Input: part model. Units: mm. Frame: model coordinates. Face numbers are marked on the shaded views. A direction names the side the tool comes from. Round coordinates to 2 decimals unless told otherwise and drop trailing zeros. Order: outer loops, then holes, each group sorted by start corner. A loop starts at its lowest first (then second) coordinate and runs counter-clockwise, first axis right, second up. Notation, with made-up numbers: (33.5, -38) -> (41.5, -38) arc R6 cw to (41.5, -30) -> close; hole circle Ø6 at (6, -32.5). An arc over 180 degrees is marked (long way). Use a Markdown table: item, result.
from build123d import *

# Parameters (mm, degrees)
SKETCH_1_W      = 23
SKETCH_1_H      = 15
SKETCH_1_R      = 1.6
EXTRUDE_1_DEPTH = 1.6
SKETCH_2_W      = 8
SKETCH_2_H      = 4
EXTRUDE_2_DEPTH = 1.8
SKETCH_4_W      = 8
SKETCH_4_H      = 1.25
EXTRUDE_3_DEPTH = 1.6
SKETCH_5_W      = 8
SKETCH_5_H      = 2.2
EXTRUDE_4_DEPTH = 1.2
FILLET_1_R      = 0.8
FILLET_2_R      = 3


with BuildPart() as part:
    # 草图1 → 凸台-拉伸1 (new body)
    with BuildSketch(Plane.XY):
        Rectangle(SKETCH_1_W, SKETCH_1_H)
        with Locations((-8, 0)):
            Circle(SKETCH_1_R, mode=Mode.SUBTRACT)
    extrude(amount=EXTRUDE_1_DEPTH)

    # 草图2 → 凸台-拉伸2 (add)
    with BuildSketch(Plane(origin=(0, 0, 0), x_dir=(-1, 0, 0), z_dir=(0, 0, -1))):
        with Locations((-0.023575702, 5.5)):
            Rectangle(SKETCH_2_W, SKETCH_2_H)
        with Locations((-0.023575702, -5.5)):
            Rectangle(SKETCH_2_W, SKETCH_2_H)
    extrude(amount=EXTRUDE_2_DEPTH)

    # 草图4 → 凸台-拉伸3 (add)
    with BuildSketch(Plane(origin=(0, 0, -1.8), x_dir=(-1, 0, 0), z_dir=(0, 0, -1))):
        with Locations((-0.023575702, 6.875)):
            Rectangle(SKETCH_4_W, SKETCH_4_H)
        with Locations((-0.023575702, -6.875)):
            Rectangle(SKETCH_4_W, SKETCH_4_H)
    extrude(amount=EXTRUDE_3_DEPTH)

    # 草图5 → 凸台-拉伸4 (add)
    with BuildSketch(Plane(origin=(0, 0, -3.4), x_dir=(-1, 0, 0), z_dir=(0, 0, -1))):
        with Locations((-0.023575702, 6.4)):
            Rectangle(SKETCH_5_W, SKETCH_5_H)
        with Locations((-0.023575702, -6.4)):
            Rectangle(SKETCH_5_W, SKETCH_5_H)
    extrude(amount=EXTRUDE_4_DEPTH)

    # 圆角1
    fillet_1_edges = [part.edges().sort_by_distance(p)[0] for p in [
        (0.023575702, 5.3, -4.6),
        (0.023575702, -5.3, -4.6),
    ]]
    fillet(fillet_1_edges, radius=FILLET_1_R)

    # 圆角2
    fillet_2_edges = [part.edges().sort_by_distance(p)[0] for p in [
        (-11.5, 7.5, 0.8),
        (11.5, 7.5, 0.8),
        (11.5, -7.5, 0.8),
        (-11.5, -7.5, 0.8),
    ]]
    fillet(fillet_2_edges, radius=FILLET_2_R)


solid = part.part
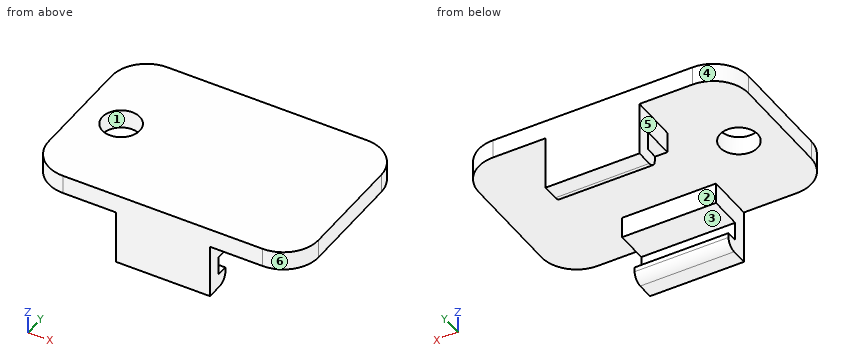
1) Set-up query: the marked faces 1 and 2. Return all of +Z, -Z, +X, -X, +Y, -Y with unobstructed straight access to the full face (end or side cutting, diameter ignored); none if empty.
Answer key:
| item | result |
|---|---|
| face 1 | +Z, -Z |
| face 2 | -Z, +X, -X |
2) Draft query along Y for the marked faces 3, 4, 5 and 6. Return one class per face: released by +Y, released by -Y, zero draft, split by the parting line, or undercut.
Answer key:
| item | result |
|---|---|
| face 3 | undercut |
| face 4 | released by +Y |
| face 5 | zero draft |
| face 6 | released by -Y |
3) Ray query, probe 1 along Y at (x, z) = (-3.5, -0.75); probe 2 along Y at (x, z) = (-8, 0.8); probe 3 along Z at (x, y) = (-9.25, -4.5). Return the intervals inside material, ascending.
Answer key:
| item | result |
|---|---|
| probe 1 | y = -7.5 to -3.5, 3.5 to 7.5 |
| probe 2 | y = -7.5 to -1.6, 1.6 to 7.5 |
| probe 3 | z = 0 to 1.6 |
4) Cut plane D-D on z = 1. Return loops of the section in (x, y).
Answer key:
| item | result |
|---|---|
| outline | (-11.5, -4.5) arc R3 ccw to (-8.5, -7.5) -> (8.5, -7.5) arc R3 ccw to (11.5, -4.5) -> (11.5, 4.5) arc R3 ccw to (8.5, 7.5) -> (-8.5, 7.5) arc R3 ccw to (-11.5, 4.5) -> close; hole circle Ø3.2 at (-8, 0) |
5) Cut plane B-B on y = 0. Return loops of the section in (x, z), and give its area (3 significant figures).
Answer key:
| item | result |
|---|---|
| outline | (-11.5, 0) -> (-9.6, 0) -> (-9.6, 1.6) -> (-11.5, 1.6) -> close; (-6.4, 0) -> (11.5, 0) -> (11.5, 1.6) -> (-6.4, 1.6) -> close |
| area | 31.7 mm^2 |
6) Cut plane A-A on z = -2.5. Return loops of the section in (x, y), and give its area (3 significant figures).
Answer key:
| item | result |
|---|---|
| outline | (-3.98, -7.5) -> (4.02, -7.5) -> (4.02, -6.25) -> (-3.98, -6.25) -> close; (-3.98, 6.25) -> (4.02, 6.25) -> (4.02, 7.5) -> (-3.98, 7.5) -> close |
| area | 20.0 mm^2 |
7) Cut plane C-C on x = 1. Return loops of the section in (y, z).
Answer key:
| item | result |
|---|---|
| outline | (-7.5, -4.6) -> (-6.1, -4.6) arc R0.8 ccw to (-5.3, -3.8) -> (-5.3, -3.4) -> (-6.25, -3.4) -> (-6.25, -1.8) -> (-3.5, -1.8) -> (-3.5, 0) -> (3.5, 0) -> (3.5, -1.8) -> (6.25, -1.8) -> (6.25, -3.4) -> (5.3, -3.4) -> (5.3, -3.8) arc R0.8 ccw to (6.1, -4.6) -> (7.5, -4.6) -> (7.5, 1.6) -> (-7.5, 1.6) -> close |
8) Contact query for flat-ended pins moving along their axis: P1, Ø1.5, axis at y = -5.5, z = 0, coming from the -X side; P2, Ø2, axis at x = 6, y = 0.5, coming from the -Z side; P3, Ø3, axis at y = -5.5, z = -2.5, coming from the +X side. Output: stop coordinate, or through.
Answer key:
| item | result |
|---|---|
| P1 | stops at x = -11.49 |
| P2 | stops at z = 0 |
| P3 | stops at x = 4.02 |
